from build123d import *

# Parameters (mm, degrees)
ESQUISSE1_W            = 33
ESQUISSE1_H            = 30
BOSS_EXTRU_1_DEPTH     = 3
D_GAGEMENT_M1_61_D     = 2.6
D_GAGEMENT_M1_61_DEPTH = 50


with BuildPart() as part:
    # Esquisse1 → Boss.-Extru.1 (new body)
    with BuildSketch(Plane.XY):
        Rectangle(ESQUISSE1_W, ESQUISSE1_H)
    extrude(amount=BOSS_EXTRU_1_DEPTH)

    # Dégagement M1.61
    with Locations(Plane.XY.offset(3)):
        with Locations((-14.036286849, -12.486010391)):
            Hole(D_GAGEMENT_M1_61_D / 2, depth=D_GAGEMENT_M1_61_DEPTH)


solid = part.part
The listing builds one solid part. Answer for the finished solid, in the listing's coordinates (mm). Give positions to 0.01 mm unless a question says otherwise; leave off trailing zeros. Write each loop counter-clockwise with the first axis right and the second up, starting at its lowest first coordinate (ties: lowest second). Pieces come first, ordered by that corner, then holes.
1) Find the intervals of material crossed by L1, parallel to X at y = -13.5, z = 2.45, in increasing order.
2) Section A-A (y = -12) is taken. Write down the section's boundary in (x, z), and give its area (3 significant figures).
3) For a pull along X with two mould halves and no side action, classify faces 1 (the face through (0, 0, 0)), 2 (the face through (-12.738, -12.429, 1.479)), 3 (the face through (16.5, 0, 1)), 4 (the face through (-16.5, 0, 1)) as pulls with the +X half, pulls with the -X half, needs draft (parallel to the pull), parting line crosses it, or undercut.
Response:
1. L1: x = -16.5 to -14.85, -13.22 to 16.5
2. outline: (-16.5, 0) - (-15.24, 0) - (-15.24, 3) - (-16.5, 3) - close; (-12.83, 0) - (16.5, 0) - (16.5, 3) - (-12.83, 3) - close
2. area: 91.8 mm2
3. face 1: needs draft
3. face 2: undercut
3. face 3: pulls with the +X half
3. face 4: pulls with the -X half
